from build123d import *

# Parameters (mm, degrees)
BOSS_EXTRUDE1_DEPTH = 11.5951
CUT_EXTRUDE4_DEPTH  = 31.957976501
SKETCH4_R           = 1.143
CUT_EXTRUDE5_DEPTH  = 30.935473315


with BuildPart() as part:
    # Sketch1 → Boss-Extrude1 (new body)
    with BuildSketch(Plane(origin=(0, 0, 0), x_dir=(1, 0, 0), z_dir=(0, 1, 0))):
        Polygon((0, 0), (7.1755, 0), (7.1755, -10.0203), (18.9865, -10.0203), (18.9865, 0), (26.162, 0), (26.162, -3.0226), (20.5994, -3.0226), (20.5994, -11.811), (5.5626, -11.811), (5.5626, -3.0226), (0, -3.0226), align=None)
    extrude(amount=BOSS_EXTRUDE1_DEPTH)

    # Sketch2 → Cut-Extrude4 (cut, through all)
    with BuildSketch(Plane.XY.offset(11.811)):
        with BuildLine():
            Line((5.5626, 8.509), (5.5626, 11.5951))
            Line((5.5626, 11.5951), (0, 11.5951))
            Line((0, 11.5951), (0, 4.318))
            ThreePointArc((0, 4.318), (1.22751548, 7.28148452), (4.191, 8.509))
            Line((4.191, 8.509), (5.5626, 8.509))
        make_face()
        with BuildLine():
            ThreePointArc((4.191, 0), (1.22751548, 1.22751548), (0, 4.191))
            Line((0, 4.191), (0, 0))
            Line((0, 0), (4.191, 0))
        make_face()
        with BuildLine():
            Line((26.162, 11.5951), (20.5994, 11.5951))
            Line((20.5994, 11.5951), (20.5994, 8.509))
            Line((20.5994, 8.509), (21.971, 8.509))
            ThreePointArc((21.971, 8.509), (24.93448452, 7.28148452), (26.162, 4.318))
            Line((26.162, 4.318), (26.162, 11.5951))
        make_face()
        with BuildLine():
            Line((26.162, 0), (26.162, 4.191))
            ThreePointArc((26.162, 4.191), (24.93448452, 1.22751548), (21.971, 0))
            Line((21.971, 0), (26.162, 0))
        make_face()
    extrude(amount=-CUT_EXTRUDE4_DEPTH, mode=Mode.SUBTRACT)

    # Sketch4 → Cut-Extrude5 (cut, through all)
    with BuildSketch(Plane.XY.offset(3.0226)):
        with Locations((4.191, 4.2545)):
            Circle(SKETCH4_R)
        with Locations((21.971, 4.2545)):
            Circle(SKETCH4_R)
    extrude(amount=-CUT_EXTRUDE5_DEPTH, mode=Mode.SUBTRACT)


solid = part.part
The listing builds one solid part. Answer for the finished solid, in the listing's coordinates (mm). A direction names the side the tool comes from. Give positions to 0.01 mm unless a question says otherwise; leave off trailing zeros. Order: outer loops, then holes, each group sorted by start corner. A loop starts at its lowest first (then second) coordinate and runs counter-clockwise, first axis right, second up. Notation, with made-up numbers: (75, 21) - (107, 21) arc R21 cw to (107, 43) - close; hole circle Ø10 at (52, 87.25). An arc over 180 degrees is marked (long way). One line per item, written item: value. Start each with the question number.
1) Find the intervals of material crossed by L1, parallel to X at y = 0.5, z = 3.25; L2, parallel to Y at x = 4.25, z = 1.25; L3, parallel to Z at x = 17.5, y = 10.75, in increasing order.
2) A cutting plane is placed at D-D on x = 9.25. Give the vertices of the cut face in (y, z), then the cut area to 3 significant figures.
3) A cutting plane is placed at B-B on z = 6. Give the vertices of the cut face in (x, y).
4) A cutting plane is placed at C-C on y = 10.5. Give the vertices of the cut face in (x, z), then the cut area to 4 significant figures.
5) The mould has two halves that part along Y. Classify faces 1 (the face through (5, 8.509, 2)), 2 (the face through (24.967, 1.26, 1.532)), 3 (the face through (23.06, 4.6, 1.53)): released by +Y, released by -Y, zero draft, split by the parting line, or undercut.
6) Given pin 1 Ø1.7 at (x, y) = (3.5, 5) entering from +Z; pin 2 Ø1.5 at (y, z) = (10, 10.5) entering from -X; pin 3 Ø6 at (y, z) = (6, 8) entering from +X, each flat-ended and moving along its own axis, determine where each tip first touches the part or whether it passes through.
7) A tool of negligible diameter and unlimited length cuts with its end or side. For faces 4 (the face through (2.8, 4.2, 3.023)), 5 (the face through (23.4, 4.2, 3.023)), 6 (the face through (13, 6, 10.02)), 7 (the face through (21, 8.509, 2)), from which of +Z, -Z, +X, -X, +Y, -Y can it reach the whole face along a straight path? Write none if from no direction.
8) A cutting plane is placed at A-A on z = 2.25. Give the vertices of the cut face in (x, y), then the cut area to 3 significant figures.
Answer sheet:
1. L1: x = 5.56 to 7.18, 18.99 to 20.6
1. L2: y = 0 to 3.11, 5.4 to 8.51
1. L3: z = 10.02 to 11.81
2. outline: (0, 10.02) - (11.6, 10.02) - (11.6, 11.81) - (0, 11.81) - close
2. area: 20.8 mm2
3. outline: (5.56, 0) - (7.18, 0) - (7.18, 11.6) - (5.56, 11.6) - close; (18.99, 0) - (20.6, 0) - (20.6, 11.6) - (18.99, 11.6) - close
4. outline: (5.56, 0) - (7.18, 0) - (7.18, 10.02) - (18.99, 10.02) - (18.99, 0) - (20.6, 0) - (20.6, 11.81) - (5.56, 11.81) - close
4. area: 59.25 mm2
5. face 1: released by +Y
5. face 2: released by -Y
5. face 3: undercut
6. pin 1: stops at z = 3.02
6. pin 2: stops at x = 5.56
6. pin 3: stops at x = 20.6
7. face 4: +Z, -X, +Y, -Y
7. face 5: +Z, +X, +Y, -Y
7. face 6: -Z, +Y, -Y
7. face 7: +Z, -Z, +X, +Y
8. outline: (0, 4.19) arc R4.19 ccw to (4.19, 0) - (7.18, 0) - (7.18, 11.6) - (5.56, 11.6) - (5.56, 8.51) - (4.19, 8.51) arc R4.19 ccw to (0, 4.32) - close; (18.99, 0) - (21.97, 0) arc R4.19 ccw to (26.16, 4.19) - (26.16, 4.32) arc R4.19 ccw to (21.97, 8.51) - (20.6, 8.51) - (20.6, 11.6) - (18.99, 11.6) - close; hole circle Ø2.29 at (4.19, 4.25); hole circle Ø2.29 at (21.97, 4.25)
8. area: 109 mm2
